Can you work these out from the drawing? Everything is in mm from the part's minimum corner. Coordinates: 2 decimals unless noted, no trailing zeros. Use a Markdown table: item, result. Add a question column.
Item 1: Will this pin go through, and if not, where does the flat tip stop? pin 1 Ø2 at (y, z) = (147.5, 16) entering from +X.
Item 2: Imagine slicing it at A-A, the plane y = 71.5. Count the separate pieces of the cut face and the enclosed holes in it, and give its area (3 significant figures).
Item 3: If I drill on line 1 along X through (y, z) = (185, 45.5); line 2 along X through (y, z) = (123, 98); line 3 along X through (y, z) = (95.5, 6), over which ranges is the centre line in solid material (lowest first)? Write a range as from..to.
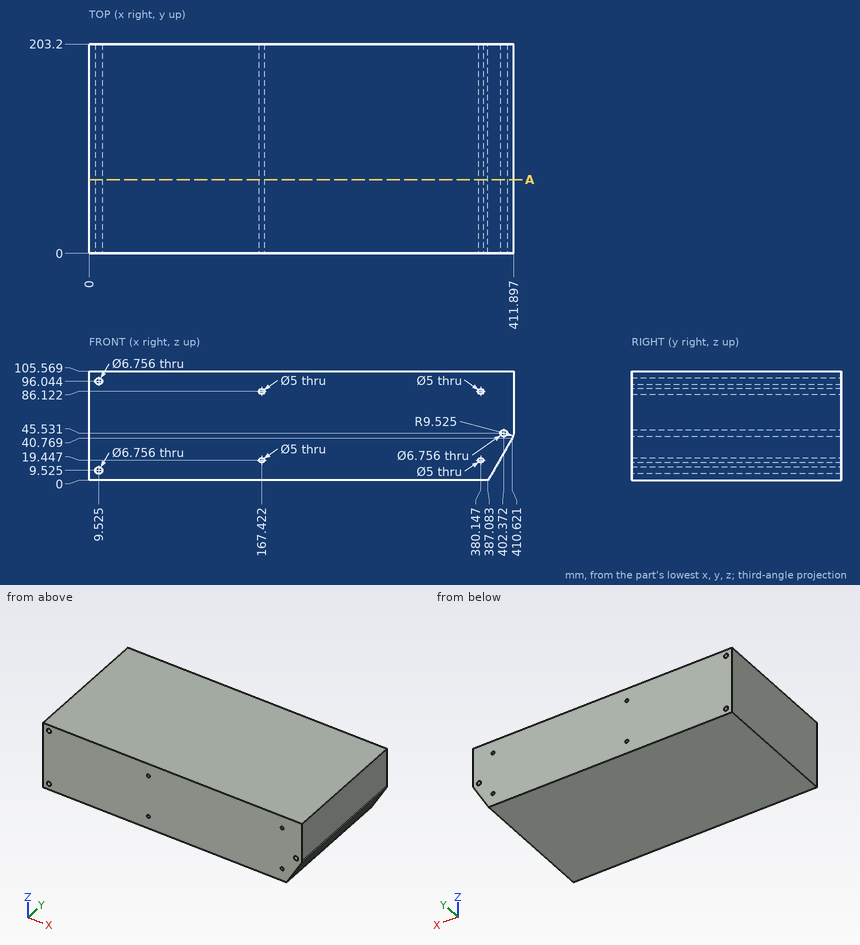
Ans:
| question | item | result |
|---|---|---|
| 1 | pin 1 | stops at x = 396.9 |
| 2 | separate pieces | 1 |
| 2 | enclosed holes | 7 |
| 2 | area | 42,800 mm^2 |
| 3 | line 1 | x = 0..398.99, 405.75..411.9 |
| 3 | line 2 | x = 0..6.77, 12.28..411.9 |
| 3 | line 3 | x = 0..390.55 |
